The drawing under review shows one solid part. Ordinate dimensions are in mm from its lowest x, y, z. A direction names the side the tool comes from. Give positions to 0.01 mm unless a question says otherwise; leave off trailing zeros. Write each loop counter-clockwise with the first axis right and the second up, starting at its lowest first coordinate (ties: lowest second). Pieces come first, ordered by that corner, then holes. Notation, with made-up numbers: (-17.75, 51.25) -> (33.25, 51.25) arc R15 cw to (33.25, 68.25) -> close; hole circle Ø1 at (37.25, -33). An arc over 180 degrees is marked (long way). Answer as a JSON object with one key per item and string values.
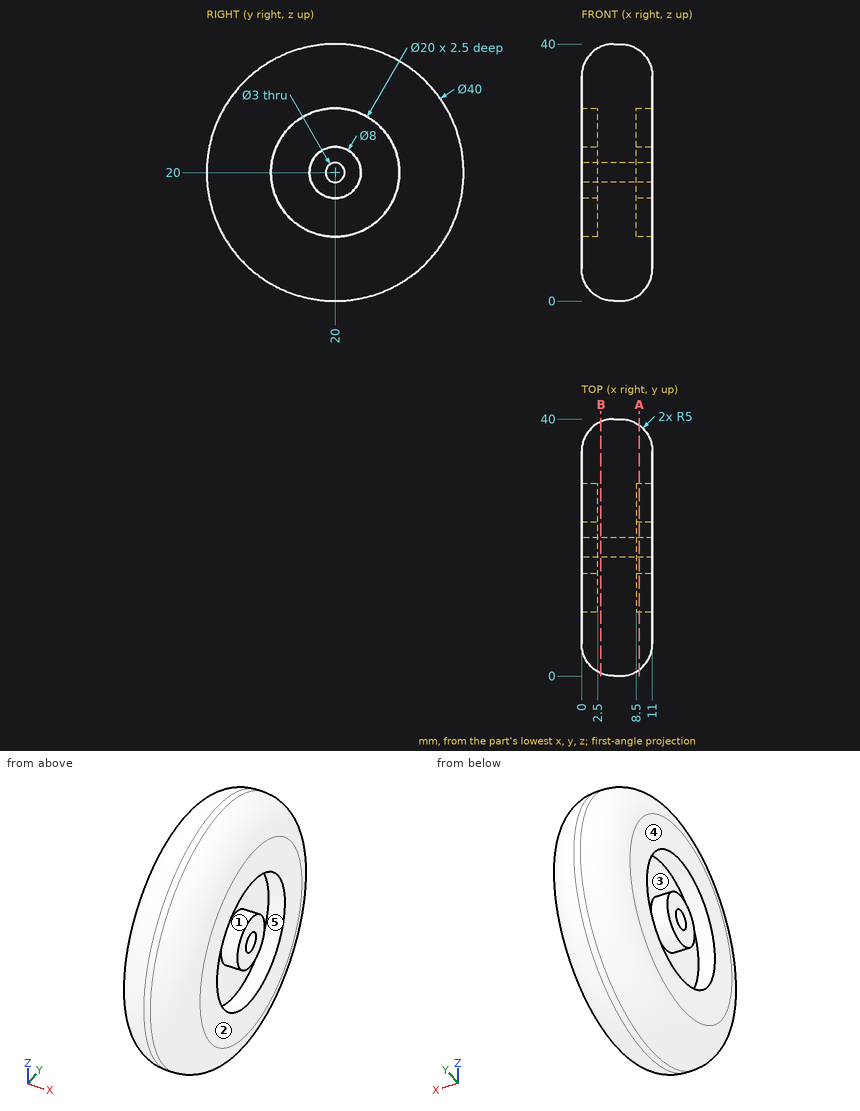
(1) For the marked faces 1, 2 and 3, list the 3-axis set-ups (+Z, -Z, +X, -X, +Y, -Y) from which the entire face can be reached by the end or side of a thin tool; tool diameter is ignored.
Here are the results:
{"face 1": "+X", "face 2": "+Z, -Z, +X, +Y, -Y", "face 3": "-X"}
(2) Clearance check with flat-ended pins moving along their axes: pin 1 (10 mm diameter, centred on y = 18.5, z = 17.5, fed in from -X); pin 2 (6 mm diameter, centred on x = 6, z = 26, fed in from +Y); pin 3 (1.8 mm diameter, centred on y = 20, z = 20, fed in from -X); pin 4 (1.5 mm diameter, centred on y = 27.5, z = 23, fed in from +X). State where each tip first meets the part, or that it passes through.
Here are the results:
{"pin 1": "stops at x = 0", "pin 2": "stops at y = 39.77", "pin 3": "passes through", "pin 4": "stops at x = 8.5"}
(3) For line 1 along Y through (x, z) = (10.05, 20); line 2 along Y through (x, z) = (3, 20); line 3 along X through (y, z) = (34, 14), list the stretches that pass through material, from the lowest coordinate up.
Here are the results:
{"line 1": "y = 2.07 to 10, 16 to 18.5, 21.5 to 24, 30 to 37.93", "line 2": "y = 0.42 to 18.5, 21.5 to 39.58", "line 3": "x = 0.01 to 10.99"}
(4) The part is to be moulded in two halves that separate along Z. For the marked faces 4 and 5, say which applies: +Z half, -Z half, draft (parallel to the pull), parting line (faces both ways), or undercut.
Here are the results:
{"face 4": "draft", "face 5": "undercut"}
(5) We need section A-A, the plane x = 9. State the section outline as (y, z) points, then the cut area to 3 significant figures.
Here are the results:
{"outline": "circle Ø38 at (20, 20); circle Ø8 at (20, 20); hole circle Ø20 at (20, 20); hole circle Ø3 at (20, 20)", "area": "863 mm²"}
(6) We need section B-B, the plane x = 3. State the section outline as (y, z) points.
Here are the results:
{"outline": "circle Ø39.17 at (20, 20); hole circle Ø3 at (20, 20)"}
